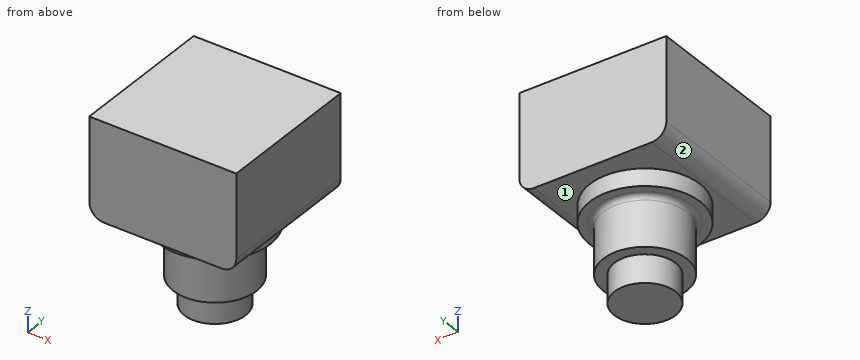
Autodesk Inventor part; units mm, degrees
ref_plane "YZ Plane" through (0, 0, 0) normal (1, 0, 0) x (0, 1, 0)
ref_plane "XZ Plane" through (0, 0, 0) normal (0, 1, 0) x (-1, 0, 0)
ref_plane "XY Plane" through (0, 0, 0) normal (0, 0, 1) x (1, 0, 0)
sketch "Boceto1" plane through (0, 0, 0) normal (0, 1, 0) x (-1, 0, 0)
  line L0 (0, 0) -> (-60, 0)
  line L1 (-60, 0) -> (-60, -34)
  line L2 (-54, -40) -> (-6, -40)
  line L3 (0, -34) -> (0, 0)
  arc A0 (-6, -40) -> (0, -34) centre (-6, -34) ccw
  arc A1 (-60, -34) -> (-54, -40) centre (-54, -34) ccw
  point P0 (-60, -40)
  dimension "d0" = 60
  dimension "d1" = 40
  dimension "d2" = 6
  dimension "d3" = 6
extrude "Extrusión1" add sketch "Boceto1" along normal blind 60
sketch "Boceto2" plane through (54, 0, -40) normal (0, 0, -1) x (-1, 0, 0)
  line L0 (0, 0) -> (48, 0)
  line L1 (48, 0) -> (48, 60)
  line L2 (0, 60) -> (48, 60)
  line L3 (0, 0) -> (0, 60)
  circle A0 centre (24, 30) radius 22.5
  circle A1 centre (24, 30) radius 17
  circle A2 centre (24, 30) radius 15
  circle A3 centre (24, 30) radius 12.5
  point P0 (54, 0)
  dimension "d6" = 45
  dimension "d7" = 34
  dimension "d8" = 30
  dimension "d9" = 25
extrude "Extrusión3" add sketch "Boceto2" along normal blind 7 contours A0
sketch "Boceto5" plane through (30, 30, -40) normal (0, 0, -1) x (-1, 0, 0)
  circle A0 centre (0, 0) radius 17
  point P0 (30, -30)
  dimension "d14" = 34
extrude "Extrusión4" add sketch "Boceto5" along normal blind 27.59
fillet "Empalme1" radius 2 1 edges at (47, 30, -47)
sketch "Boceto8" plane through (30, 30, -67.59) normal (0, 0, -1) x (-1, 0, 0)
  circle A0 centre (0, 0) radius 12.5
  point P0 (30, -30)
  dimension "d23" = 25
extrude "Extrusión6" add sketch "Boceto8" along normal blind 11.41
sketch "Boceto9" plane through (30, 30, -79) normal (0, 0, -1) x (-1, 0, 0)
  point P0 (30, -30)
equation "\"Radio_pliegue\" = Grosor"
equation "\"Anchura_desahogo_plegado\" = Grosor"
equation "\"Profundidad_desahogo_plegado\" = 0.5 * Grosor"
equation "\"Tamaño_destalonado\" = 4 * Grosor"
equation "\"Remanente_mínimo\" = 2 * Grosor"
equation "\"Radiodetransición\" = Radio_pliegue"
equation "\"Tamaño_de_radio_de_Jacobi\" = Radio_pliegue"
equation "\"TamañoSeparación\" = Grosor"
properties part number "Practica 12 nt"
Can you work these out from the model? Positions are in its coordinate system, mm. Face numbers are marked on the shaded views. A direction names the side the tool comes from. Give positions to 0.01 mm unless a question says otherwise; leave off trailing zeros. Loops run counter-clockwise (first coordinate to the right, second up) from the corner with the lowest first, then second, coordinate; pieces in that order, holes last. Notation, with made-up numbers: M -26,67.5 L 14,67.5 A25 cw 14,101.5 Z; hole C 68,42.5 d7. An arc over 180 degrees is marked long. Use one line per item in the form item = value. Start each with the question number.
(1) I want a section at B-B, the plane y = 30. Write out the boundary of the cut face in (x, z).
(2) I want a section at D-D, the plane y = 4.5. Write out the boundary of the cut face in (x, z).
(3) On a 3-axis mill with a long thin cutter (end or side, diameter ignored), from which of +Z, -Z, +X, -X, +Y, -Y can I reach the whole of each face in a straight line? I mean the marked faces 1 and 2. Say none if no direction works.
(4) I want a section at A-A, the plane x = 30. Write out the boundary of the cut face in (y, z), and give its area (3 significant figures).
(5) I want a section at C-C, the plane z = -41. Write out the boundary of the cut face in (x, y), and give its area (3 significant figures).
(6) I'm going to push flat-ended pins straight in: P1, Ø6, axis at y = 39, z = -40, coming from the +X side; P2, Ø3, axis at x = 18.5, z = -51.5, coming from the +Y side; P3, Ø5, axis at x = 34.5, z = -66, coming from the -Y side. Where does each tip first touch, or does it pass through?
(7) Please list where these lines run through material, in increasing order: line 1 (Z direction, x = 20.5, y = 7.5); line 2 (Z direction, x = 32, y = 8); line 3 (Y direction, x = 30, z = -73).
Worked out:
q1.outline = M 0,-34 A6 ccw 6,-40 L 7.5,-40 L 7.5,-47 L 11,-47 A2 cw 13,-49 L 13,-67.59 L 17.5,-67.59 L 17.5,-79 L 42.5,-79 L 42.5,-67.59 L 47,-67.59 L 47,-49 A2 cw 49,-47 L 52.5,-47 L 52.5,-40 L 54,-40 A6 ccw 60,-34 L 60,0 L 0,0 Z
q2.outline = M 0,-34 A6 ccw 6,-40 L 54,-40 A6 ccw 60,-34 L 60,0 L 0,0 Z
q3.face_1 = -Z
q3.face_2 = -Z, -X, +Y, -Y
q4.outline = M 0,-40 L 7.5,-40 L 7.5,-47 L 11,-47 A2 cw 13,-49 L 13,-67.59 L 17.5,-67.59 L 17.5,-79 L 42.5,-79 L 42.5,-67.59 L 47,-67.59 L 47,-49 A2 cw 49,-47 L 52.5,-47 L 52.5,-40 L 60,-40 L 60,0 L 0,0 Z
q4.area = 3,700 mm²
q5.outline = C 30,30 d45
q5.area = 1,590 mm²
q6.P1 = 59.2
q6.P2 = 43.75
q6.P3 = 13.12
q7.line_1 = -40 to 0
q7.line_2 = -47 to 0
q7.line_3 = 17.5 to 42.5
